from build123d import *

# Parameters (mm, degrees)
BOSS_EXTRUDE1_DEPTH = 15


with BuildPart() as part:
    # Sketch1 → Boss-Extrude1 (new body)
    with BuildSketch(Plane(origin=(-154.007123162, 0, 0), x_dir=(0, -1, 0), z_dir=(-1, 0, 0))):
        with BuildLine():
            Line((-657.135362842, -373.543546556), (-660.3297369, -367.554095198))
            ThreePointArc((-660.3297369, -367.554095198), (-660.508248633, -367.366340196), (-660.757920333, -367.297185139))
            Line((-660.757920333, -367.297185139), (-669.463950035, -367.297185139))
            ThreePointArc((-669.463950035, -367.297185139), (-669.713621735, -367.366340196), (-669.892133468, -367.554095198))
            Line((-669.892133468, -367.554095198), (-673.086507526, -373.543546556))
            ThreePointArc((-673.086507526, -373.543546556), (-665.110935184, -386.836167126), (-657.135362842, -373.543546556))
        make_face()
        with BuildLine():
            Line((-672.169758714, -374.032479256), (-669.110935184, -368.297185139))
            Line((-669.110935184, -368.297185139), (-661.110935184, -368.297185139))
            Line((-661.110935184, -368.297185139), (-658.052111655, -374.032479256))
            ThreePointArc((-658.052111655, -374.032479256), (-665.110935184, -385.797185139), (-672.169758714, -374.032479256))
        make_face(mode=Mode.SUBTRACT)
    extrude(amount=-BOSS_EXTRUDE1_DEPTH)


solid = part.part
Part model, mm, in its own coordinate system. A direction names the side the tool comes from. Coordinates: 2 decimals unless noted, no trailing zeros. Order: outer loops, then holes, each group sorted by start corner. A loop starts at its lowest first (then second) coordinate and runs counter-clockwise, first axis right, second up.
(1) Slice it at C-C, the plane y = 668.75. Write the cut outline in (x, z), and give its area (3 significant figures).
Check sheet entries:
outline: (-154.01, -386.07) - (-139.01, -386.07) - (-139.01, -384.92) - (-154.01, -384.92) - close; (-154.01, -368.3) - (-139.01, -368.3) - (-139.01, -367.3) - (-154.01, -367.3) - close
area: 32.2 mm2
(2) Slice it at A-A, the plane z = -377. Write the cut outline in (x, y), and give its area (3 significant figures).
Check sheet entries:
outline: (-154.01, 656.11) - (-139.01, 656.11) - (-139.01, 657.15) - (-154.01, 657.15) - close; (-154.01, 673.07) - (-139.01, 673.07) - (-139.01, 674.11) - (-154.01, 674.11) - close
area: 31.3 mm2
(3) Tool access for faces 1 (the face through (-147, 665, -368.297)), 2 (the face through (-154.007, 672, -373)): list every direction of +Z, -Z, +X, -X, +Y, -Y with a clear straight run to the whole face (end or side of a thin tool).
Check sheet entries:
face 1: +X, -X
face 2: +Z, -Z, -X, +Y, -Y
(4) Pull direction Z, two halves, no side cores. Call faces 3 (the face through (-146.612, 665.372, -386.832)), 4 (the face through (-139.007, 672, -373)), 5 (the face through (-146.61, 671.47, -370.51)), 6 (the face through (-146.612, 659.603, -371.125)): pulls with the +Z half, pulls with the -Z half, needs draft (parallel to the pull), parting line crosses it, or undercut.
Check sheet entries:
face 3: parting line crosses it
face 4: needs draft
face 5: pulls with the +Z half
face 6: undercut
(5) Slice it at B-B, the plane x = -143.25. Write the cut outline in (y, z).
Check sheet entries:
outline: (657.14, -373.54) arc R9.04 ccw (long way) to (673.09, -373.54) - (669.89, -367.55) arc R0.49 ccw to (669.46, -367.3) - (660.76, -367.3) arc R0.49 ccw to (660.33, -367.55) - close; hole (658.05, -374.03) arc R8 ccw (long way) to (672.17, -374.03) - (669.11, -368.3) - (661.11, -368.3) - close
(6) Pin check, flat tips, straight feed: pin 1 Ø2 at (x, z) = (-149, -376.5) entering from -Y; pin 2 Ø1 at (x, z) = (-151, -374.5) entering from -Y; pin 3 Ø4 at (x, y) = (-152.5, 662.5) entering from -Z. Stop position of each tip, or through.
Check sheet entries:
pin 1: stops at y = 656.08
pin 2: stops at y = 656.52
pin 3: stops at z = -386.82
(7) Probe L1, parallel to Y at x = -141.75, z = -385; L2, parallel to Z at x = -149.25, y = 669; L3, parallel to Z at x = -144, y = 666. List the from-to ranges inside material, lowest first.
Check sheet entries:
L1: y = 659.65 to 661.63, 668.59 to 670.57
L2: z = -385.96 to -384.79, -368.3 to -367.3
L3: z = -386.79 to -385.75, -368.3 to -367.3
